from build123d import *

# Parameters (mm, degrees)
BOSS_EXTRUDE1_DEPTH = 3
SKETCH2_W           = 221
SKETCH2_H           = 357.28000224
BOSS_EXTRUDE2_DEPTH = 3


with BuildPart() as part:
    # Sketch1 → Boss-Extrude1 (new body)
    with BuildSketch(Plane(origin=(107.5, 0, 0), x_dir=(0, 0, -1), z_dir=(1, 0, 0))):
        Polygon((125.5, 330), (-131.5, 330), (-231.5, -13), (125.5, -13), align=None)
    extrude(amount=BOSS_EXTRUDE1_DEPTH)


with BuildPart() as body_2:
    # Mirror2: mirrored copy
    add(part.part.mirror(Plane(origin=(0, 0, 0), x_dir=(0, 0, 1), z_dir=(1, 0, 0))))


with BuildPart() as part_1:
    add(part.part)

    add(body_2.part)  # Boss-Extrude2 merges body 2
    # Sketch2 → Boss-Extrude2 (add)
    with BuildSketch(Plane(origin=(0, 61.18692665, 209.871158411), x_dir=(1, 0, 0), z_dir=(0, 0.27989252, 0.960031342))):
        with Locations((0, 101.364475406)):
            Rectangle(SKETCH2_W, SKETCH2_H)
    extrude(amount=BOSS_EXTRUDE2_DEPTH)


solid = part_1.part
Work out the finished part from the listing and answer in its coordinate system (mm). A direction names the side the tool comes from. Give positions to 0.01 mm unless a question says otherwise; leave off trailing zeros. Loops run counter-clockwise (first coordinate to the right, second up) from the corner with the lowest first, then second, coordinate; pieces in that order, holes last. Notation, with made-up numbers: (-37.75, -6.75) -> (18.25, -6.75) arc R10 ccw to (18.25, -2.75) -> close; hole circle Ø7 at (-27.75, 86.25). An arc over 180 degrees is marked (long way). Use a Markdown table: item, result. Add a question column.
1. Find the intervals of material crossed by probe 1 along X at (y, z) = (245, 130); probe 2 along Z at (x, y) = (55, 17.5); probe 3 along Z at (x, y) = (66, 108), in increasing order.
2. Determine the mould class of faces 1 (the flat face through (-1.55, 161.74, 183.68)), 2 (the flat face through (110.5, 153, 44)), 3 (the flat face through (107.5, 161, 16)) for opening direction X: released by +X, released by -X, zero draft, split by the parting line, or undercut.
3. Section B-B on y = 108 is taken. Determine the outline of the cut face in (x, z).
4. Section A-A on z = -32.5 is taken. Determine the outline of the cut face in (x, y), and give its area (3 significant figures).
5. Section D-D on z = 141 is taken. Determine the outline of the cut face in (x, y) (3 decimals).
6. Flat-ended cylindrical pins translate along their axes: pin 1 Ø1.5 at (x, z) = (109, -39) entering from +Y; pin 2 Ø1 at (x, y) = (-18.5, 243) entering from -Z. Find the tip coordinate at first contact, or state that the pin passes through.
7. Section C-C on x = -22.5 is taken. Determine the outline of the cut face in (y, z), and give its area (3 significant figures).
8. For faces 4 (the flat face through (-107.5, 161, 16)), 5 (the flat face through (-110.5, 153, 44)), determine the directions among +Z, -Z, +X, -X, +Y, -Y from which every point of the face is accessible in a straight line to the end or side of a thin tool.
Results below:
| question | item | result |
|---|---|---|
| 1 | probe 1 | x = -110.5 to -107.5, 107.5 to 110.5 |
| 1 | probe 2 | z = 222.61 to 225.73 |
| 1 | probe 3 | z = 196.22 to 199.35 |
| 2 | face 1 | zero draft |
| 2 | face 2 | released by +X |
| 2 | face 3 | undercut |
| 3 | outline | (-110.5, -125.5) -> (-107.5, -125.5) -> (-107.5, 196.22) -> (107.5, 196.22) -> (107.5, -125.5) -> (110.5, -125.5) -> (110.5, 199.35) -> (-110.5, 199.35) -> close |
| 4 | outline | (-110.5, -13) -> (-107.5, -13) -> (-107.5, 330) -> (-110.5, 330) -> close; (107.5, -13) -> (110.5, -13) -> (110.5, 330) -> (107.5, 330) -> close |
| 4 | area | 2,060 mm^2 |
| 5 | outline | (-110.5, -13) -> (-107.5, -13) -> (-107.5, 297.415) -> (107.5, 297.415) -> (107.5, -13) -> (110.5, -13) -> (110.5, 308.133) -> (-110.5, 308.133) -> close |
| 6 | pin 1 | stops at y = 330 |
| 6 | pin 2 | stops at z = 156.72 |
| 7 | outline | (-13, 231.5) -> (330, 131.5) -> (330.84, 134.38) -> (-12.16, 234.38) -> close |
| 7 | area | 1,070 mm^2 |
| 8 | face 4 | -Z, -Y |
| 8 | face 5 | +Z, -Z, -X, +Y, -Y |
